```python
from build123d import *

# Parameters (mm, degrees)
CROQUIS1_R              = 2.25
SALIENTE_EXTRUIR2_DEPTH = 15
CROQUIS2_W              = 8
CROQUIS2_H              = 30
CORTAR_EXTRUIR1_DEPTH   = 1
CROQUIS5_R              = 28
CORTAR_EXTRUIR2_DEPTH   = 5.5
CHAFL_N1_SIZE           = 4
CROQUIS6_W              = 27
CROQUIS6_H              = 4
CORTAR_EXTRUIR3_DEPTH   = 62.686708544
CROQUIS7_W              = 21
CROQUIS7_H              = 1.5
CORTAR_EXTRUIR4_DEPTH   = 62.686708455
CORTAR_EXTRUIR5_REACH   = 60.568
CROQUIS8_W              = 8
CROQUIS8_H              = 9.5
CHAFL_N2_SIZE           = 6
CHAFL_N3_SIZE           = 0.5
CROQUIS9_R              = 3.5
CORTAR_EXTRUIR6_DEPTH   = 42.800119617
CROQUIS10_R             = 4
CORTAR_EXTRUIR7_DEPTH   = 19.5


with BuildPart() as part:
    # Croquis1 → Saliente-Extruir2 (new body)
    with BuildSketch(Plane(origin=(0, 0, 0), x_dir=(1, 0, 0), z_dir=(0, 1, 0))):
        with BuildLine():
            Line((3, 20), (24.839745962, 20))
            Line((24.839745962, 20), (33.5, 15))
            Line((33.5, 15), (44.5, 15))
            Line((44.5, 15), (44.5, -15))
            Line((44.5, -15), (33.5, -15))
            Line((33.5, -15), (24.839745962, -20))
            Line((24.839745962, -20), (3, -20))
            Line((3, -20), (3, -16.479153498))
            ThreePointArc((3, -16.479153498), (16.75, 0), (3, 16.479153498))
            Line((3, 16.479153498), (3, 20))
        make_face()
        with Locations(Location((40.5, 10, 0), (0, 0, 270))):
            Circle(CROQUIS1_R, mode=Mode.SUBTRACT)
        with Locations(Location((40.5, -10, 0), (0, 0, 270))):
            Circle(CROQUIS1_R, mode=Mode.SUBTRACT)
    extrude(amount=SALIENTE_EXTRUIR2_DEPTH)

    # Croquis2 → Cortar-Extruir1 (cut)
    with BuildSketch(Plane(origin=(0, 15, 0), x_dir=(1, 0, 0), z_dir=(0, 1, 0))):
        with Locations((40.5, 0)):
            Rectangle(CROQUIS2_W, CROQUIS2_H)
    extrude(amount=-CORTAR_EXTRUIR1_DEPTH, mode=Mode.SUBTRACT)

    # Croquis3 → Cortar-Revolución1 (revolve, cut)
    with BuildSketch(Plane.XY):
        Polygon((16.75, 0), (16.75, 1), (17.327350269, 0), align=None)
    revolve(axis=Axis((0, 15, 0), (0, -1, 0)), mode=Mode.SUBTRACT)

    # Croquis5 → Cortar-Extruir2 (cut)
    with BuildSketch(Plane(origin=(0, 15, 0), x_dir=(1, 0, 0), z_dir=(0, 1, 0))):
        Circle(CROQUIS5_R)
    extrude(amount=-CORTAR_EXTRUIR2_DEPTH, mode=Mode.SUBTRACT)

    # Chaflán1
    chafl_n1_edges = [part.edges().sort_by_distance(p)[0] for p in [
        (28, 15, 0),
    ]]
    chamfer(chafl_n1_edges, length=CHAFL_N1_SIZE)

    # Croquis6 → Cortar-Extruir3 (cut, through all)
    with BuildSketch(Plane.XY.offset(20)):
        with Locations((13.5, 13)):
            Rectangle(CROQUIS6_W, CROQUIS6_H)
    extrude(amount=-CORTAR_EXTRUIR3_DEPTH, mode=Mode.SUBTRACT)

    # Croquis7 → Cortar-Extruir4 (cut, through all)
    with BuildSketch(Plane.XY.offset(20)):
        with Locations((10.5, 10.25)):
            Rectangle(CROQUIS7_W, CROQUIS7_H)
    extrude(amount=-CORTAR_EXTRUIR4_DEPTH, mode=Mode.SUBTRACT)

    # Croquis8 → Cortar-Extruir5 (cut, up to next)
    with BuildSketch(Plane.XY.offset(15), mode=Mode.PRIVATE) as cortar_extruir5_sk1:
        with Locations((40.5, 4.75)):
            Rectangle(CROQUIS8_W, CROQUIS8_H)
    cortar_extruir5_tool1 = extrude(cortar_extruir5_sk1.sketch, amount=-CORTAR_EXTRUIR5_REACH, mode=Mode.PRIVATE) & part.part
    add(cortar_extruir5_tool1.solids().sort_by_distance((40.5, 4.75, 15))[0], mode=Mode.SUBTRACT)

    # Chaflán2
    chafl_n2_edges = [part.edges().sort_by_distance(p)[0] for p in [
        (36.5, 0, 0),
    ]]
    chamfer(chafl_n2_edges, length=CHAFL_N2_SIZE)

    # Chaflán3
    chafl_n3_edges = [part.edges().sort_by_distance(p)[0] for p in [
        (16.75, 9.5, 0),
    ]]
    chamfer(chafl_n3_edges, length=CHAFL_N3_SIZE)

    # Croquis9 → Cortar-Extruir6 (cut, through all)
    with BuildSketch(Plane(origin=(36.5, 0, 0), x_dir=(0, 0, -1), z_dir=(1, 0, 0))):
        with Locations((0, 5)):
            Circle(CROQUIS9_R)
    extrude(amount=-CORTAR_EXTRUIR6_DEPTH, mode=Mode.SUBTRACT)

    # Croquis10 → Cortar-Extruir7 (cut)
    with BuildSketch(Plane(origin=(36.5, 0, 0), x_dir=(0, 0, -1), z_dir=(1, 0, 0))):
        with Locations((0, 5)):
            Circle(CROQUIS10_R)
    extrude(amount=-CORTAR_EXTRUIR7_DEPTH, mode=Mode.SUBTRACT)


solid = part.part
```
Can you work these out from the model? Positions are in its coordinate system, mm. A direction names the side the tool comes from. Coordinates: 2 decimals unless noted, no trailing zeros. Loops run counter-clockwise (first coordinate to the right, second up) from the corner with the lowest first, then second, coordinate; pieces in that order, holes last.
Item 1: I'm going to push flat-ended pins straight in: pin 1 (0.8 mm diameter, centred on y = 14.5, z = 2, fed in from +X); pin 2 (5 mm diameter, centred on y = 5, z = 0, fed in from -X) (3 decimals); pin 3 (5 mm diameter, centred on x = 23, z = 13, fed in from +Y); pin 4 (4 mm diameter, centred on x = 41, z = -5, fed in from -Y). Where does each tip first touch, or does it pass through?
Answers below:
pin 1: stops at x = 36.5
pin 2: passes through
pin 3: stops at y = 11
pin 4: stops at y = 9.5
Item 2: Suppose I cut it at D-D (x = 40.5). Please give me the cut outline in (y, z), then the cut area to 3 significant figures.
Answers below:
outline: (9.5, -15) - (14, -15) - (14, -12.25) - (9.5, -12.25) - close; (9.5, -7.75) - (14, -7.75) - (14, 7.75) - (9.5, 7.75) - close; (9.5, 12.25) - (14, 12.25) - (14, 15) - (9.5, 15) - close
area: 94.5 mm2
Item 3: Suppose I cut it at A-A (z = 0). Please give me the cut outline in (x, y), then the cut area to 3 significant figures.
Answers below:
outline: (16.75, 1) - (17.33, 0) - (30.5, 0) - (31.5, 1) - (17, 1) - (17, 1.5) - (16.75, 1.5) - close; (16.75, 8.5) - (17, 8.5) - (17, 9) - (36.5, 9) - (36.5, 9.5) - (44.5, 9.5) - (44.5, 14) - (36.5, 14) - (36.5, 15) - (32, 15) - (28, 11) - (28, 9.5) - (17.25, 9.5) - (16.75, 9) - close
area: 98.7 mm2
Item 4: Suppose I cut it at B-B (y = 5). Please give me the cut outline in (x, z).
Answers below:
outline: (3, -20) - (24.84, -20) - (33.5, -15) - (35.5, -15) - (35.5, -4) - (17, -4) - (17, -3.5) - (16.38, -3.5) arc R16.75 cw to (3, -16.48) - close; (3, 16.48) arc R16.75 cw to (16.38, 3.5) - (17, 3.5) - (17, 4) - (35.5, 4) - (35.5, 15) - (33.5, 15) - (24.84, 20) - (3, 20) - close
Item 5: Which directions (+Z, -Z, +X, -X, +Y, -Y) give clear straight access to the entire face, cutting with the end or side of a thin tool? Please do faces 4 (the face through (25, 11, 17)), 5 (the face through (18, 9.5, 0)), 6 (the face through (38, 10, 15)).
Answers below:
face 4: +Z, -Z, -X, +Y
face 5: -X, +Y
face 6: +Z, +X, +Y, -Y
Item 6: Suppose I cut it at C-C (y = 10.25). Please give me the cut outline in (x, z), then the cut area to 3 significant figures.
Answers below:
outline: (21, -20) - (24.84, -20) - (33.5, -15) - (44.5, -15) - (44.5, 15) - (33.5, 15) - (24.84, 20) - (21, 20) - (21, 18.52) arc R28 cw to (21, -18.52) - close; hole circle Ø4.5 at (40.5, -10); hole circle Ø4.5 at (40.5, 10)
area: 577 mm2
Item 7: If we mould it in two halves opening along X, with no side actions, what happens to faces 1 (the face through (42.73, 11.72, 9.71)), 2 (the face through (29.109, 7.395, -17.535)), 3 (the face through (33, 15, 0))? For each: released by +X, released by -X, zero draft, split by the parting line, or undercut.
Answers below:
face 1: undercut
face 2: released by +X
face 3: zero draft
Item 8: Please list where these lines run through material, in increasing order: L1, parallel to Z at x = 40.5, y = 12.25; L2, parallel to Z at x = 16.9, y = 5; L3, parallel to Y at x = 27, z = 0.
Answers below:
L1: z = -15 to -12.25, -7.75 to 7.75, 12.25 to 15
L2: z = -20 to -3.5, 3.5 to 20
L3: y = 0 to 1, 9 to 9.5
